Autodesk Inventor part; units mm, degrees
ref_plane "YZ Plane" through (0, 0, 0) normal (1, 0, 0) x (0, 1, 0)
ref_plane "XZ Plane" through (0, 0, 0) normal (0, 1, 0) x (-1, 0, 0)
ref_plane "XY Plane" through (0, 0, 0) normal (0, 0, 1) x (1, 0, 0)
sketch "Sketch1" plane through (0, 0, 0) normal (0, 0, 1) x (1, 0, 0)
  line L0 (10, -10) -> (-10, -10)
  line L1 (-10, -10) -> (-10, 10)
  line L2 (-10, 10) -> (10, 10)
  line L3 (10, 10) -> (10, -10)
  line L4 (10, -10) -> (-10, 10) construction
  line L5 (-10, -10) -> (10, 10) construction
  line L6 (10, -10) -> (6, -10)
  line L7 (6, -10) -> (6, 10)
  line L8 (6, 10) -> (10, 10)
  line L9 (10, 10) -> (10, -10)
  line L10 (6, 2) -> (4, 2)
  line L11 (4, 2) -> (4, -2)
  line L12 (4, -2) -> (6, -2)
  line L13 (6, -2) -> (6, 2)
  line L14 (0, 10) -> (0, -10)
  point P0 (0, 0)
  dimension "d0" = 20
  dimension "d1" = 20
  dimension "d2" = 4
  dimension "d6" = 2
  dimension "d7" = 2
  dimension "d8" = 4
  dimension "d9" = 2
extrude "Extrusion1" add sketch "Sketch1" along normal blind 5 contours L0 L14 L2 L7 L10 L11 L12
ref_plane "Work Plane1" through (0, 0, 2.5) normal (0, 0, 1) x (1, 0, 0)
sketch "Sketch2" plane through (0, 0, 2.5) normal (0, 0, 1) x (1, 0, 0)
  line L0 (0, 10) -> (0, -10)
  line L1 (0, 3.1754) -> (2.75, 1.5877)
  line L2 (2.75, 1.5877) -> (2.75, -1.5877)
  line L3 (2.75, -1.5877) -> (0, -3.1754)
  line L4 (0, -3.1754) -> (-2.75, -1.5877)
  line L5 (-2.75, -1.5877) -> (-2.75, 1.5877)
  line L6 (-2.75, 1.5877) -> (0, 3.1754)
  point P0 (0, 0)
  point P1 (0, 0)
  dimension "d12" = 5.5
extrude "Extrusion2" cut sketch "Sketch2" along normal mid plane 1.8
sketch "Sketch3" plane through (0, 0, 5) normal (0, 0, 1) x (1, 0, 0)
  circle A0 centre (0, 0) radius 1.75
  dimension "d15" = 3.5
extrude "Extrusion3" cut sketch "Sketch3" against normal blind 8
sketch "Sketch4" plane through (0, 10, 0) normal (-1, 0, 0) x (0, 0, 1)
  circle A0 centre (2.5, -2.5) radius 0.8
  circle A1 centre (2.5, -17.5) radius 0.8
  line L0 (0, 0) -> (5, 0)
  line L1 (0, 0) -> (0, -8.25)
  line L2 (0, -11.75) -> (0, -20)
  line L3 (0, -20) -> (5, -20)
  point P0 (0, -10)
  dimension "d18" = 1.6
  dimension "d19" = 1.6
  dimension "d20" = 2.5
  dimension "d21" = 2.5
  dimension "d22" = 2.5
  dimension "d23" = 2.5
extrude "Extrusion4" cut sketch "Sketch4" against normal blind 5
thread "Thread1"
thread "Thread2"
sketch "Sketch5" plane through (0, 0, 0) normal (0, 0, -1) x (-1, 0, 0)
  line L0 (-6, -2) -> (-4, -2)
  line L1 (-4, -2) -> (-6, -2)
  line L2 (-6, -2) -> (-6, 2)
  line L3 (-6, 2) -> (-4, 2)
  line L4 (-4, 2) -> (-4, -2)
  point P0 (0, 0)
extrude "Extrusion5" add sketch "Sketch5" against normal blind 5
sketch "Sketch6" plane through (0, 0, 0) normal (0, 0, -1) x (-1, 0, 0)
  line L0 (-6, -10) -> (-6, 10)
  circle A0 centre (-6, 6) radius 2.5
  line L1 (-6, -9) -> (-3.5, -9)
  line L2 (-3.5, -9) -> (-3.5, -3)
  line L3 (-3.5, -3) -> (-6, -3)
  line L4 (-6, -3) -> (-6, -9)
  line L5 (0, -10) -> (-6, -10)
  line L6 (-6, 10) -> (0, 10)
  point P0 (0, 0)
  dimension "d32" = 2.5
  dimension "d33" = 1
  dimension "d34" = 6
  dimension "d35" = 5
  dimension "d36" = 4
extrude "Extrusion6" cut sketch "Sketch6" against normal blind 5
sketch "Sketch7" plane through (6, -3, 0) normal (1, 0, 0) x (0, 0, -1)
  circle A0 centre (-2.5, 3) radius 1.1
  line L0 (0, 0) -> (0, 6.5)
  line L1 (0, -7) -> (-5, -7)
  point P0 (0, 3)
  dimension "d39" = 2.5
  dimension "d40" = 10
  dimension "d41" = 2.2
extrude "Extrusion7" cut sketch "Sketch7" against normal blind 20
equation "\"d19\" = d18"
properties part number "POMSliderMotor"
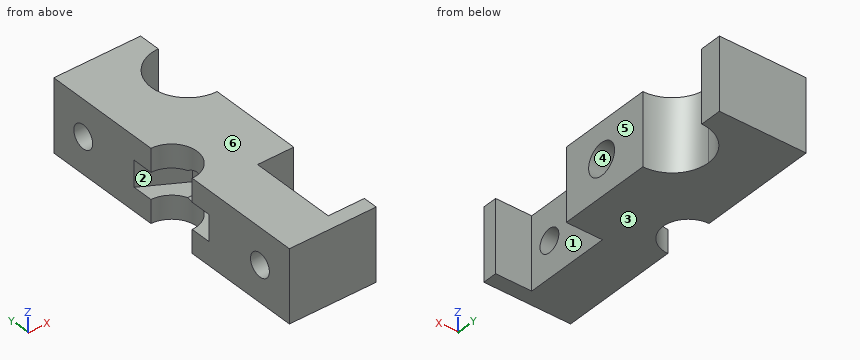
The model under review builds one solid part; all positions refer to its coordinate system, in mm. Face numbers are marked on the shaded views. A direction names the side the tool comes from. Round coordinates to 2 decimals unless told otherwise and drop trailing zeros. Order: outer loops, then holes, each group sorted by start corner. A loop starts at its lowest first (then second) coordinate and runs counter-clockwise, first axis right, second up.
Item 1: Add section D-D, the plane x = 2. State the section outline as (y, z) points, and give its area (3 significant figures).
Working result:
outline: (-10, 0) - (10, 0) - (10, 5) - (-10, 5) - close; hole circle Ø1.6 at (-7.5, 2.5); hole (-2.02, 1.6) - (-0.63, 1.6) arc R1.1 ccw to (0.63, 1.6) - (2.02, 1.6) - (2.02, 3.4) - (0.63, 3.4) arc R1.1 ccw to (-0.63, 3.4) - (-2.02, 3.4) - close; hole circle Ø1.6 at (7.5, 2.5)
area: 88.4 mm2
Item 2: Add section B-B, the plane x = 5.5. State the section outline as (y, z) points.
Working result:
outline: (-10, 0) - (-9, 0) - (-9, 5) - (-10, 5) - close; (-3, 0) - (3.55, 0) - (3.55, 5) - (-3, 5) - close; (8.45, 0) - (10, 0) - (10, 5) - (8.45, 5) - close; hole circle Ø2.2 at (0, 2.5)
Item 3: Draft analysis for pull direction Z (two halves, no side actions). For the marked faces 4, 5 and 6, state which applies: released by +Z, released by -Z, zero draft, split by the parting line, or undercut.
Working result:
face 4: undercut
face 5: zero draft
face 6: released by +Z
Item 4: To check wall thickness, follow probe 1 along Y at (x, z) = (3.1, 2.5); probe 2 along Z at (x, y) = (3.45, 0); probe 3 along Y at (x, z) = (4.35, 2.5). State the ranges of each line that lie inside material, in increasing order.
Working result:
probe 1: y = -10 to -8.3, -6.7 to -1.1, 1.1 to 6.7, 8.3 to 10
probe 2: z = 0 to 1.4, 3.6 to 5
probe 3: y = -10 to -9, -3 to -1.1, 1.1 to 4.12, 8.3 to 10
Item 5: Machinability: for the marked faces 1, 2 and 3, which of the approach directions +Z, -Z, +X, -X, +Y, -Y give a long, thin tool a straight path to every point of the face, cutting with its end or side? Answer none if there is none.
Working result:
face 1: +Z, -Z, +X
face 2: -X
face 3: -Z, +X, -X, +Y, -Y
Item 6: Add section C-C, the plane z = 0.8. State the section outline as (x, y) points.
Working result:
outline: (0, -10) - (6, -10) - (6, -9) - (3.5, -9) - (3.5, -3) - (6, -3) - (6, 3.5) arc R2.5 cw to (6, 8.5) - (6, 10) - (0, 10) - (0, 1.75) arc R1.75 cw to (0, -1.75) - close
Item 7: Add section A-A, the plane y = 0. State the section outline as (x, z) points, and give its area (3 significant figures).
Working result:
outline: (1.75, 0) - (6, 0) - (6, 1.4) - (1.75, 1.4) - close; (1.75, 3.6) - (6, 3.6) - (6, 5) - (1.75, 5) - close
area: 11.9 mm2
Item 8: For pin 1 (1.4 mm diameter, centred on y = 7.5, z = 2.5, fed in from +X); pin 2 (0.8 mm diameter, centred on y = -1, z = 2.5, fed in from -X), all flat-tipped, find the tip position at first contact; note any pin that passes through.
Working result:
pin 1: passes through
pin 2: stops at x = 2.75
